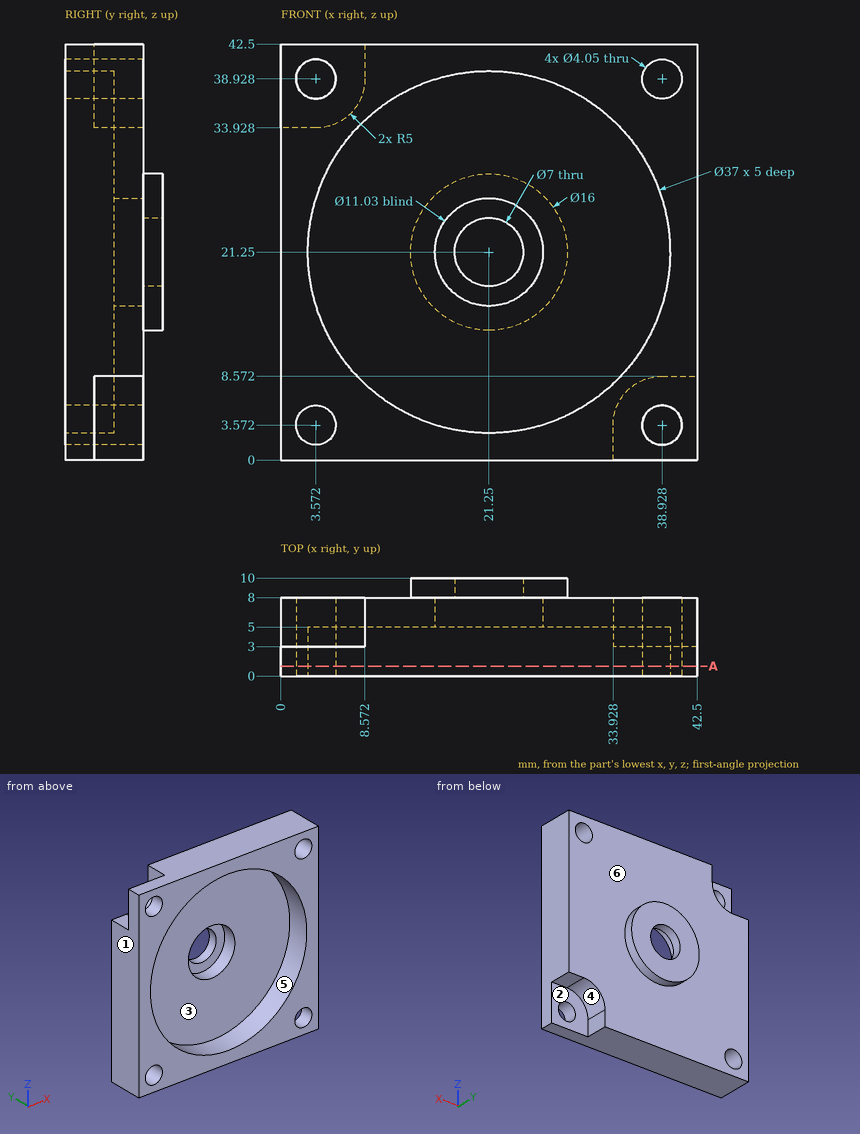
For this review, use the dimensioned drawing (mm, ordinates from the lowest corner) and the shaded views. A direction names the side the tool comes from. Coordinates: 2 decimals unless noted, no trailing zeros.
1. Add section A-A, the plane y = 1. Count the separate pieces of the cut face and the enclosed holes in it.
2. Mouldability with a two-part tool opening along Z and no side actions: class the marked faces 4, 5 and 6 as +Z half, -Z half, draft (parallel to the pull), parting line (faces both ways), or undercut.
3. For line 1 (X direction, y = 8.8, z = 21.25); line 2 (X direction, y = 5.9, z = 21.25) (1 decimal); line 3 (Y direction, x = 15, z = 24), list the stretches that pass through material, from the lowest coordinate up.
4. For the marked faces 1, 2 and 3, list the 3-axis set-ups (+Z, -Z, +X, -X, +Y, -Y) from which the entire face can be reached by the end or side of a thin tool; tool diameter is ignored.
5. Insertion check: P1, Ø6, axis at x = 22, z = 9.5, coming from the -Y side; P2, Ø3, axis at y = 5, z = 1.5, coming from the +X side; P3, Ø7, axis at x = 3.5, z = 40, coming from the +Y side. Each pin has a flat end and moves straight along its axis. Give the tip position at first contact, or say it passes through.
Result:
1. separate pieces: 1
1. enclosed holes: 5
2. face 4: -Z half
2. face 5: undercut
2. face 6: draft
3. line 1: x = 13.25 to 17.75, 24.75 to 29.25
3. line 2: x = 0 to 15.7, 26.8 to 42.5
3. line 3: y = 5 to 10
4. face 1: +Z, -Z, -X, +Y, -Y
4. face 2: -Z, +X, +Y
4. face 3: -Y
5. P1: stops at y = 5
5. P2: stops at x = 33.93
5. P3: stops at y = 3
